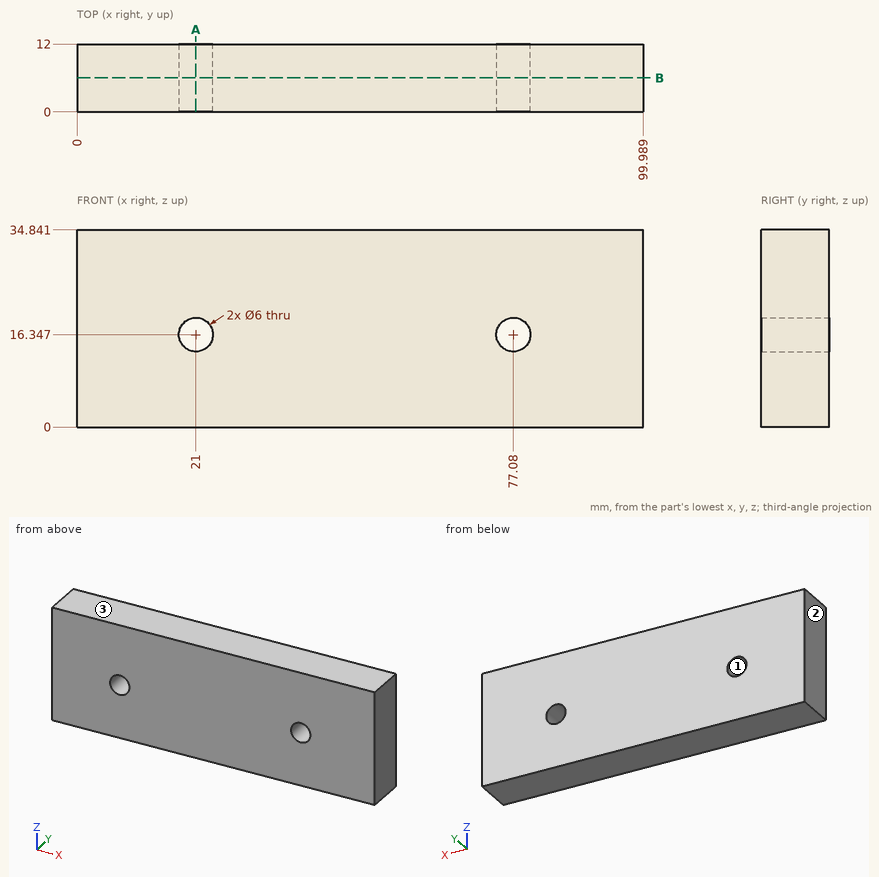
Source: three-view drawing plus pictorial views. Frame: mm from the lowest corner of the part. Coordinates: 2 decimals unless noted, no trailing zeros. Order: outer loops, then holes, each group sorted by start corner. A loop starts at its lowest first (then second) coordinate and runs counter-clockwise, first axis right, second up. Notation, with made-up numbers: (-15, 78) -> (1, 78) arc R4 ccw to (1, 84) -> close; hole circle Ø8 at (-12.75, -9). An arc over 180 degrees is marked (long way). Write item = value, one per line.
(1) Cut plane A-A on x = 21. Return loops of the section in (y, z).
Solved:
outline = (0, 0) -> (12, 0) -> (12, 13.35) -> (0, 13.35) -> close; (0, 19.35) -> (12, 19.35) -> (12, 34.84) -> (0, 34.84) -> close
(2) Pin query (flat end, axial travel): pin 1 Ø9.5 at (x, z) = (77.08, 16.35) entering from -Y. Return the tip coordinate at first contact, or that it passes through.
Solved:
pin_1 = 0
(3) Cut plane B-B on y = 6. Return loops of the section in (x, z), plus the area to 3 significant figures.
Solved:
outline = (0, 0) -> (99.99, 0) -> (99.99, 34.84) -> (0, 34.84) -> close; hole circle Ø6 at (21, 16.35); hole circle Ø6 at (77.08, 16.35)
area = 3,430 mm²
(4) Line query: line 1 (Z direction, x = 21, y = 9); line 2 (Z direction, x = 78.5, y = 6) (1 decimal). Output: solid intervals per line, ascending.
Solved:
line_1 = 0 to 13.35, 19.35 to 34.84
line_2 = 0 to 13.7, 19 to 34.8
(5) Pull-direction query (X, two-part tool) for the marked faces 1, 2 and 3; classes: pulls with the +X half, pulls with the -X half, needs draft (parallel to the pull), parting line crosses it, or undercut.
Solved:
face_1 = undercut
face_2 = pulls with the -X half
face_3 = needs draft
